from build123d import *

# Parameters (mm, degrees)
ESQUISSE1_W                                = 200
ESQUISSE1_H                                = 160
ESQUISSE1_R                                = 5
ESQUISSE1_R_2                              = 1.75
ESQUISSE1_W_2                              = 10
ESQUISSE1_H_2                              = 10
ESQUISSE1_H_3                              = 30
BOSS_EXTRU_1_DEPTH                         = 5
CONG_2_R                                   = 1
ENL_V_MAT_EXTRU_1_DEPTH                    = 129.16005618
ESQUISSE3_R                                = 1.75
TROU_CUVE_DIRECTION_DEPTH                  = 129.16005618
ESQUISSE4_R                                = 1.7
ESQUISSE4_R_2                              = 4
ESQUISSE4_R_3                              = 5
POINTE_AVANT_TROUS_BERCEAU_ET_CABLES_DEPTH = 129.16005618


with BuildPart() as part:
    # Esquisse1 → Boss.-Extru.1 (new body)
    with BuildSketch(Plane(origin=(0, 0, 0), x_dir=(0, 1, 0), z_dir=(0, 0, 1))):
        Rectangle(ESQUISSE1_W, ESQUISSE1_H)
        with Locations(Location((-75, 0, 0), (0, 0, 270))):
            Circle(ESQUISSE1_R, mode=Mode.SUBTRACT)
        with Locations(Location((-57.5, 35.5, 0), (0, 0, 270))):
            Circle(ESQUISSE1_R_2, mode=Mode.SUBTRACT)
        with Locations(Location((-57.5, -35.5, 0), (0, 0, 90))):
            Circle(ESQUISSE1_R_2, mode=Mode.SUBTRACT)
        with Locations(Location((65, 45, 0), (0, 0, 270))):
            Circle(ESQUISSE1_R_2, mode=Mode.SUBTRACT)
        with Locations(Location((65, -45, 0), (0, 0, 90))):
            Circle(ESQUISSE1_R_2, mode=Mode.SUBTRACT)
        with Locations(Location((-31, 37.5, 0), (0, 0, 270))):
            Circle(ESQUISSE1_R_2, mode=Mode.SUBTRACT)
        with Locations(Location((-31, 75, 0), (0, 0, 270))):
            Circle(ESQUISSE1_R_2, mode=Mode.SUBTRACT)
        with Locations(Location((6.5, 75, 0), (0, 0, 270))):
            Circle(ESQUISSE1_R_2, mode=Mode.SUBTRACT)
        with Locations(Location((6.5, 37.5, 0), (0, 0, 270))):
            Circle(ESQUISSE1_R_2, mode=Mode.SUBTRACT)
        with Locations(Location((-31, -46.541307377, 0), (0, 0, 270))):
            Circle(ESQUISSE1_R_2, mode=Mode.SUBTRACT)
        with Locations(Location((-31, -70.091307377, 0), (0, 0, 270))):
            Circle(ESQUISSE1_R_2, mode=Mode.SUBTRACT)
        with Locations(Location((15.5, -46.541307377, 0), (0, 0, 270))):
            Circle(ESQUISSE1_R_2, mode=Mode.SUBTRACT)
        with Locations(Location((15.5, -70.091307377, 0), (0, 0, 270))):
            Circle(ESQUISSE1_R_2, mode=Mode.SUBTRACT)
        with Locations(Location((-4.999283545, 0, 0), (0, 0, 270))):
            Circle(ESQUISSE1_R_2, mode=Mode.SUBTRACT)
        with Locations(Location((85, 33, 0), (0, 0, 270))):
            Circle(ESQUISSE1_R_2, mode=Mode.SUBTRACT)
        with Locations(Location((85.001189598, -32.999999989, 0), (0, 0, 270))):
            Circle(ESQUISSE1_R_2, mode=Mode.SUBTRACT)
        with Locations(Location((19, 33, 0), (0, 0, 270))):
            Circle(ESQUISSE1_R_2, mode=Mode.SUBTRACT)
        with Locations(Location((19.001189598, -32.999999989, 0), (0, 0, 270))):
            Circle(ESQUISSE1_R_2, mode=Mode.SUBTRACT)
        with Locations((-46, 35)):
            Rectangle(ESQUISSE1_W_2, ESQUISSE1_H_2, mode=Mode.SUBTRACT)
        with Locations((7, 0)):
            Rectangle(ESQUISSE1_W_2, ESQUISSE1_H_3, mode=Mode.SUBTRACT)
    extrude(amount=BOSS_EXTRU_1_DEPTH)

    # Congé2
    cong_2_edges = [part.edges().sort_by_distance(p)[0] for p in [
        (-40, -51, 2.5),
        (-30, -51, 2.5),
        (-30, -41, 2.5),
        (-40, -41, 2.5),
        (-15, 2, 2.5),
        (15, 2, 2.5),
        (15, 12, 2.5),
        (-15, 12, 2.5),
    ]]
    fillet(cong_2_edges, radius=CONG_2_R)

    # Esquisse2 → Enlèv. mat.-Extru.1 (cut, through all)
    with BuildSketch(Plane.XY.offset(5)):
        Polygon((-573.580399643, 598.167108478), (-698.698151963, -488.082468479), (684.299979338, -647.380682556), (762.904681953, 702.431902078), align=None)
        Polygon((-110, 40), (0, 160), (110, 40), (110, -40), (0, -160), (-110, -40), align=None, mode=Mode.SUBTRACT)
    extrude(amount=-ENL_V_MAT_EXTRU_1_DEPTH, mode=Mode.SUBTRACT)

    # Esquisse3 → Trou cuve direction (cut, through all)
    with BuildSketch(Plane(origin=(0, 0, 0), x_dir=(0, 1, 0), z_dir=(0, 0, 1))):
        with Locations(Location((-94.001515359, 0.004041019, 0), (0, 0, 270))):
            Circle(ESQUISSE3_R)
    extrude(amount=TROU_CUVE_DIRECTION_DEPTH, mode=Mode.SUBTRACT)

    # Esquisse4 → Pointe avant, trous berceau et cables (cut, through all)
    with BuildSketch(Plane.XY.offset(5)):
        with Locations((-63.004041019, 23.738484641)):
            Circle(ESQUISSE4_R)
        with Locations((-63.004041019, 41.738484641)):
            Circle(ESQUISSE4_R)
        with Locations((62.995958981, 23.738484641)):
            Circle(ESQUISSE4_R)
        with Locations((62.995958981, 41.738484641)):
            Circle(ESQUISSE4_R)
        with Locations((-63.004041019, 32.738484641)):
            Circle(ESQUISSE4_R_2)
        with Locations((62.995958981, 32.738484641)):
            Circle(ESQUISSE4_R_2)
        with Locations((-24.724041019, -20.261515359)):
            Circle(ESQUISSE4_R_3)
        with Locations((24.675958981, -20.261515359)):
            Circle(ESQUISSE4_R_3)
        Polygon((-82.024041019, 47.038484641), (-45.024041019, 103.038484641), (-83.024041019, 103.038484641), (-83.024041019, 47.038484641), align=None)
        Polygon((82.015958981, 47.038484641), (45.015958981, 103.038484641), (83.015958981, 103.038484641), (83.015958981, 47.038484641), align=None)
    extrude(amount=-POINTE_AVANT_TROUS_BERCEAU_ET_CABLES_DEPTH, mode=Mode.SUBTRACT)


solid = part.part
Input: part model. Units: mm. Frame: model coordinates. A direction names the side the tool comes from. Coordinates: 2 decimals unless noted, no trailing zeros. Loops run counter-clockwise (first coordinate to the right, second up) from the corner with the lowest first, then second, coordinate; pieces in that order, holes last.
Q1. Material intervals for line 1 (Y direction, x = -37.5, z = 3.1); line 2 (Y direction, x = -13, z = 3.5); line 3 (Y direction, x = 0, z = 1.7), sorted ascending.
Q2. Cut plane B-B (z = 2.95). Give the number of separate pieces and of enclosed holes in the cut face, then the cut area to 3 significant figures.
Q3. Set-up query: faces 4 (the face through (-30, -46, 2)), 5 (the face through (67.68, -86.17, 2.54)). Return all of +Z, -Z, +X, -X, +Y, -Y with unobstructed straight access to the full face (end or side cutting, diameter ignored); none if empty.
Q4. Cut plane A-A (y = -88). Output: boundary loops of the cut face in (x, z).
Q5. Draft query along X for faces 1 (the face through (-63.75, 74.7, 2.54)), 2 (the face through (0, 2, 2)), 3 (the face through (1, -100, 2)). Return one class per face: +X half, -X half, draft (parallel to the pull), parting line (faces both ways), or undercut.
Q6. Cut plane C-C (y = 58). Output: boundary loops of the cut face in (x, z).
Q7. Contact query for a flat-ended pin moving along its axis: pin 1 (1.5 mm diameter, centred on x = 48.5, z = 4, fed in from +Y). Output: stop coordinate, or through.
Working result:
1. line 1: y = -100 to -51, -41 to -32.75, -29.25 to 4.75, 8.25 to 100
1. line 2: y = -100 to 2, 12 to 100
1. line 3: y = -100 to -95.75, -92.25 to -80, -70 to -6.75, -3.25 to 2, 12 to 100
2. separate pieces: 1
2. enclosed holes: 29
2. area: 28,700 mm2
3. face 4: +Z, -Z
3. face 5: +Z, -Z, +X, -Y
4. outline: (-66, 0) - (66, 0) - (66, 5) - (-66, 5) - close
5. face 1: -X half
5. face 2: undercut
5. face 3: draft
6. outline: (-74.78, 0) - (74.77, 0) - (74.77, 5) - (-74.78, 5) - close
7. pin 1: stops at y = 98.9
